```python
from build123d import *

# Parameters (mm, degrees)
SKETCH2_W           = 170
SKETCH2_H           = 30
BOSS_EXTRUDE1_DEPTH = 40
SKETCH3_W           = 150
SKETCH3_H           = 10
CUT_EXTRUDE1_DEPTH  = 20
SKETCH4_R           = 5.789067321
CUT_EXTRUDE2_DEPTH  = 170


with BuildPart() as part:
    # Sketch2 → Boss-Extrude1 (new body)
    with BuildSketch(Plane(origin=(0, 0, 0), x_dir=(1, 0, 0), z_dir=(0, 1, 0))):
        with Locations((85, 15)):
            Rectangle(SKETCH2_W, SKETCH2_H)
    extrude(amount=BOSS_EXTRUDE1_DEPTH)

    # Sketch3 → Cut-Extrude1 (cut)
    with BuildSketch(Plane.XZ):
        with Locations((85, -15)):
            Rectangle(SKETCH3_W, SKETCH3_H)
    extrude(amount=-CUT_EXTRUDE1_DEPTH, mode=Mode.SUBTRACT)

    # Sketch4 → Cut-Extrude2 (cut)
    with BuildSketch(Plane(origin=(170, 0, 0), x_dir=(0, 0, -1), z_dir=(1, 0, 0))):
        with Locations((15, 30)):
            Circle(SKETCH4_R)
    extrude(amount=-CUT_EXTRUDE2_DEPTH, mode=Mode.SUBTRACT)


solid = part.part
```
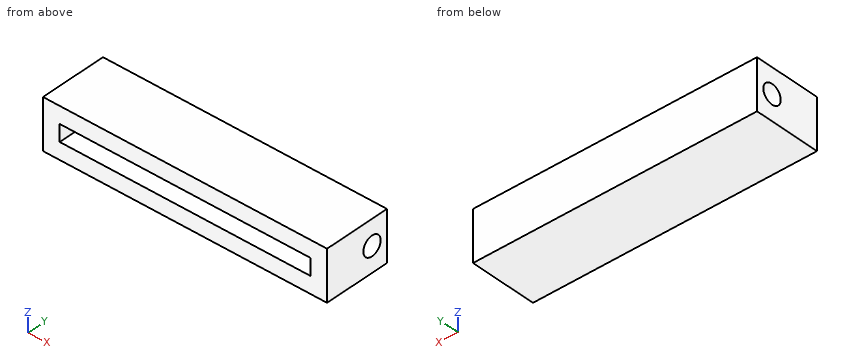
Work out the finished part from the listing and answer in its coordinate system (mm). Coordinates: 2 decimals unless noted, no trailing zeros. Write each loop counter-clockwise with the first axis right and the second up, starting at its lowest first coordinate (ties: lowest second). Pieces come first, ordered by that corner, then holes. Notation, with made-up numbers: (17.25, 25) - (45.25, 25) arc R15 ccw to (45.25, 37) - close; hole circle Ø7 at (38, 15.25). An arc over 180 degrees is marked (long way). Answer as a JSON object with one key per item and string values.
Q1. Consider L1, parallel to Y at x = 86.5, z = -15; L2, parallel to X at y = 14.5, z = -10.75; L3, parallel to Z at x = 155, y = 18. Determine where each line is inside the solid, lowest interval first. Write a range as from..to.
Results list:
{"L1": "y = 20..24.21, 35.79..40", "L2": "x = 0..10, 160..170", "L3": "z = -30..-20, -10..0"}
Q2. Find section A-A (z = -15). Write down the section's boundary in (x, y).
Results list:
{"outline": "(0, 0) - (10, 0) - (10, 20) - (160, 20) - (160, 0) - (170, 0) - (170, 24.21) - (0, 24.21) - close; (0, 35.79) - (170, 35.79) - (170, 40) - (0, 40) - close"}
Q3. Find section B-B (y = 30). Write down the section's boundary in (x, z).
Results list:
{"outline": "(0, -30) - (170, -30) - (170, -20.79) - (0, -20.79) - close; (0, -9.21) - (170, -9.21) - (170, 0) - (0, 0) - close"}
Q4. Given pin 1 Ø9.5 at (y, z) = (30, -15) entering from -X, flat-ended and moving along its own axis, determine where the tip first touches the part or whether it passes through.
Results list:
{"pin 1": "passes through"}
Q5. Find section C-C (y = 14). Write down the section's boundary in (x, z).
Results list:
{"outline": "(0, -30) - (170, -30) - (170, 0) - (0, 0) - close; hole (10, -20) - (160, -20) - (160, -10) - (10, -10) - close"}
Q6. Find section D-D (x = 127). Write down the section's boundary in (y, z), plus the area to 3 significant figures.
Results list:
{"outline": "(0, -30) - (40, -30) - (40, 0) - (0, 0) - (0, -10) - (20, -10) - (20, -20) - (0, -20) - close; hole circle Ø11.58 at (30, -15)", "area": "895 mm^2"}
